CAD build for the part. Positions are in the model's coordinates, mm. A direction names the side the tool comes from. Coordinates: 2 decimals unless noted, no trailing zeros. Write each loop counter-clockwise with the first axis right and the second up, starting at its lowest first coordinate (ties: lowest second). Pieces come first, ordered by that corner, then holes. Notation, with made-up numbers: (-1.5, 78) - (17.5, 78) arc R26 ccw to (17.5, 105) - close; hole circle Ø10 at (31.25, -30). An arc over 180 degrees is marked (long way). Answer in a Markdown table with one row per item. Add a question column.
Q1. Two-plate mould, pull along Y, no slides. Class faces 1 (the cylindrical face through (735.862, -791.867, 112.7)), 2 (the flat face through (-97, -501, 584.2)), 3 (the flat face through (-118, 0, 361)): +Y half, -Y half, draft (parallel to the pull), parting line (faces both ways), or undercut.
Q2. 3-axis set-ups, long thin cutter, end or side, ignore diameter. For faces 4 (the flat face through (-559.636, -501, 408)), 5 (the flat face through (-331.036, -501, 175)), 6 (the flat face through (354.764, -501, 405)): which of +Z, -Z, +X, -X, +Y, -Y reach the whole face in a straight line?
Q3. Band-saw the part on D-D (y = -612). List the corners of the cut face in (x, z).
Q4. Drill centre lines: line 1 along X through (y, z) = (-787, 54); line 2 along X through (y, z) = (-376, 209.5); line 3 along Y through (x, z) = (-1034, 192.5). Where is each one in solid material? Low to high. Write a range as from..to.
Q5. Pin check, flat tips, straight feed: pin 1 (1.5 mm diameter, centred on y = -470.5, z = 340, fed in from -X); pin 2 (3 mm diameter, centred on y = -198.5, z = 277.5, fed in from -X); pin 3 (1 mm diameter, centred on y = -821.5, z = 503.5, fed in from +X). Stop position of each tip, or through.
Q6. Band-saw the part on C-C (x = 839). List the corners of the cut face in (y, z), and give its area (3 significant figures).
Q7. Band-saw the part on A-A (z = 183.5). List the corners of the cut face in (x, y).
Q8. Band-saw the part on B-B (y = -228.6). List the corners of the cut face in (x, z).
```python
from build123d import *

# Parameters (mm, degrees)
F1_DEPTH = 1016
F2_R     = 50.8
F3_R     = 50.8
F4_R     = 101.6
F5_DEPTH = 228.6


# Not quite as in the source:
# - a feature names something its author has since deleted; it is built from what else it names


with BuildPart() as f1:
    # F0 (on Front) → F1 (new body)
    with BuildSketch(Plane.XZ):
        Polygon((-1270.8357659235, 228.6), (-1270.8357659235, 0), (-331.0357659235, 0), (-331.0357659235, 355.6), (126.1642340765, 355.6), (126.1642340765, 0), (1065.9642340765, 0), (1065.9642340765, 228.6), (354.7642340765, 228.6), (354.7642340765, 584.2), (-559.6357659235, 584.2), (-559.6357659235, 228.6), align=None)
    extrude(amount=F1_DEPTH)

    # F2
    f2_edges = [f1.edges().sort_by_distance(p)[0] for p in [
        (-559.635766, -508, 584.2),
        (354.764234, -508, 584.2),
        (-1270.835766, -1016, 114.3),
        (1065.964234, -1016, 114.3),
        (1065.964234, 0, 114.3),
        (-1270.835766, 0, 114.3),
    ]]
    fillet(f2_edges, radius=F2_R)

    # F3
    f3_edges = [f1.edges().sort_by_distance(p)[0] for p in [
        (354.764234, -508, 228.6),
        (-559.635766, -508, 228.6),
    ]]
    fillet(f3_edges, radius=F3_R)

    # F4 (on face) → F5 (cut)
    with BuildSketch(Plane(origin=(0, 0, 0), x_dir=(1, 0, 0), z_dir=(0, 0, -1))):
        with Locations((837.3642340765, 228.6)):
            Circle(F4_R)
        with Locations((837.3642340765, 787.4)):
            Circle(F4_R)
        with Locations((-1042.2357659235, 228.6)):
            Circle(F4_R)
        with Locations((-1042.2357659235, 787.4)):
            Circle(F4_R)
    extrude(amount=-F5_DEPTH, mode=Mode.SUBTRACT)


solid = f1.part
```
Checked values:
| question | item | result |
|---|---|---|
| 1 | face 1 | undercut |
| 1 | face 2 | draft |
| 1 | face 3 | +Y half |
| 2 | face 4 | +Z, -X, +Y, -Y |
| 2 | face 5 | -Z, +Y, -Y |
| 2 | face 6 | +Z, +X, +Y, -Y |
| 3 | outline | (-1270.84, 0) - (-331.04, 0) - (-331.04, 355.6) - (126.16, 355.6) - (126.16, 0) - (1065.96, 0) - (1065.96, 228.6) - (405.56, 228.6) arc R50.8 cw to (354.76, 279.4) - (354.76, 533.4) arc R50.8 ccw to (303.96, 584.2) - (-508.84, 584.2) arc R50.8 ccw to (-559.64, 533.4) - (-559.64, 279.4) arc R50.8 cw to (-610.44, 228.6) - (-1270.84, 228.6) - close |
| 4 | line 1 | x = -1270.84..-1143.83, -940.64..-331.04, 126.16..735.77, 938.96..1065.96 |
| 4 | line 2 | x = -1270.84..-331.04, 126.16..1065.96 |
| 4 | line 3 | y = -1016..-888.67, -686.13..-329.87, -127.33..0 |
| 5 | pin 1 | stops at x = -559.64 |
| 5 | pin 2 | stops at x = -559.75 |
| 5 | pin 3 | stops at x = 354.76 |
| 6 | outline | (-1016, 0) - (-888.99, 0) - (-888.99, 228.6) - (-1016, 228.6) - close; (-685.81, 0) - (-330.19, 0) - (-330.19, 228.6) - (-685.81, 228.6) - close; (-127.01, 0) - (0, 0) - (0, 228.6) - (-127.01, 228.6) - close |
| 6 | area | 139,000 mm² |
| 7 | outline | (-1270.84, -965.2) arc R50.8 ccw to (-1220.04, -1016) - (-331.04, -1016) - (-331.04, 0) - (-1220.04, 0) arc R50.8 ccw to (-1270.84, -50.8) - close; (126.16, -1016) - (1015.16, -1016) arc R50.8 ccw to (1065.96, -965.2) - (1065.96, -50.8) arc R50.8 ccw to (1015.16, 0) - (126.16, 0) - close; hole circle Ø203.2 at (-1042.24, -787.4); hole circle Ø203.2 at (-1042.24, -228.6); hole circle Ø203.2 at (837.36, -787.4); hole circle Ø203.2 at (837.36, -228.6) |
| 8 | outline | (-1270.84, 0) - (-1143.84, 0) - (-1143.84, 228.6) - (-1270.84, 228.6) - close; (-940.64, 0) - (-331.04, 0) - (-331.04, 355.6) - (126.16, 355.6) - (126.16, 0) - (735.76, 0) - (735.76, 228.6) - (405.56, 228.6) arc R50.8 cw to (354.76, 279.4) - (354.76, 533.4) arc R50.8 ccw to (303.96, 584.2) - (-508.84, 584.2) arc R50.8 ccw to (-559.64, 533.4) - (-559.64, 279.4) arc R50.8 cw to (-610.44, 228.6) - (-940.64, 228.6) - close; (938.96, 0) - (1065.96, 0) - (1065.96, 228.6) - (938.96, 228.6) - close |
